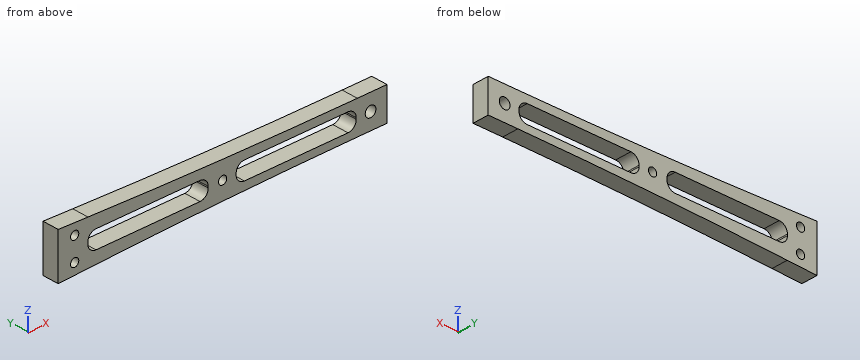
from build123d import *

# Parameters (mm, degrees)
SZKIC1_R                    = 1.97098021
SZKIC1_R_2                  = 3.25
SZKIC1_R_3                  = 2.5
DODANIE_WYCI_GNI_CIE1_DEPTH = 10
ZAOKR_GLENIE1_R             = 4100
OTW_R_GWINTOWANY_M62_D      = 5
OTW_R_GWINTOWANY_M62_DEPTH  = 15.497848452
OTW_R_GWINTOWANY_M62_TIP    = 1.502151548


with BuildPart() as part:
    # Szkic1 → Dodanie-wyciągnięcie1 (new body)
    with BuildSketch(Plane(origin=(0, 0, 0), x_dir=(1, 0, 0), z_dir=(0, 1, 0))):
        Polygon((200, 0), (200, 20), (100, 20), (0, 24), (0, -4), (100, 0), align=None)
        with Locations(Location((100, 10, 0), (0, 0, 270))):
            Circle(SZKIC1_R, mode=Mode.SUBTRACT)
        with Locations(Location((190, 10, 0), (0, 0, 270))):
            Circle(SZKIC1_R_2, mode=Mode.SUBTRACT)
        with Locations(Location((10, 17, 0), (0, 0, 270))):
            Circle(SZKIC1_R_3, mode=Mode.SUBTRACT)
        with Locations(Location((10, 3, 0), (0, 0, 270))):
            Circle(SZKIC1_R_3, mode=Mode.SUBTRACT)
        with BuildLine():
            Line((22.984822323, 15.57457628), (86.25939238, 15.57457628))
            ThreePointArc((86.25939238, 15.57457628), (89.794926286, 14.110110186), (91.25939238, 10.57457628))
            Line((91.25939238, 10.57457628), (91.25939238, 9.696719379))
            ThreePointArc((91.25939238, 9.696719379), (89.794926286, 6.161185473), (86.25939238, 4.696719379))
            Line((86.25939238, 4.696719379), (22.984822323, 4.696719379))
            ThreePointArc((22.984822323, 4.696719379), (19.449288417, 6.161185473), (17.984822323, 9.696719379))
            Line((17.984822323, 9.696719379), (17.984822323, 10.57457628))
            ThreePointArc((17.984822323, 10.57457628), (19.449288417, 14.110110186), (22.984822323, 15.57457628))
        make_face(mode=Mode.SUBTRACT)
        with BuildLine():
            Line((113.225148066, 15.57457628), (176.286209663, 15.57457628))
            ThreePointArc((176.286209663, 15.57457628), (179.821743569, 14.110110186), (181.286209663, 10.57457628))
            Line((181.286209663, 10.57457628), (181.286209663, 9.752776346))
            ThreePointArc((181.286209663, 9.752776346), (179.821743569, 6.21724244), (176.286209663, 4.752776346))
            Line((176.286209663, 4.752776346), (113.225148066, 4.752776346))
            ThreePointArc((113.225148066, 4.752776346), (109.68961416, 6.21724244), (108.225148066, 9.752776346))
            Line((108.225148066, 9.752776346), (108.225148066, 10.57457628))
            ThreePointArc((108.225148066, 10.57457628), (109.68961416, 14.110110186), (113.225148066, 15.57457628))
        make_face(mode=Mode.SUBTRACT)
    extrude(amount=DODANIE_WYCI_GNI_CIE1_DEPTH)

    # Zaokrąglenie1
    # the kernel refuses this fillet: 4100 mm, written as the material it adds along each edge
    with BuildSketch(Plane(origin=(100, 0, -20), x_dir=(1, 0, 0), z_dir=(0, 1, 0)), Plane(origin=(100, 0, 0), x_dir=(-0.9992009587217893, 0, 0.03996803834887583), z_dir=(0, 1, 0))) as zaokr_glenie1_piece_1:
        with BuildLine():
            CenterArc((ZAOKR_GLENIE1_R * 0.0199920063936, ZAOKR_GLENIE1_R), ZAOKR_GLENIE1_R, 267.709389957, 2.290610043)
            Line((-ZAOKR_GLENIE1_R * 0.0199760319553, ZAOKR_GLENIE1_R * 0.000799041278211), (0, 0))
            Line((0, 0), (ZAOKR_GLENIE1_R * 0.0199920063936, 0))
        make_face()
    extrude(amount=10)

    # Otwór gwintowany M62
    with Locations(Plane(origin=(100, 10, -10), x_dir=(0, 0, 1), z_dir=(0, 1, 0))):
        with Locations((0, 0)):
            Hole(OTW_R_GWINTOWANY_M62_D / 2, depth=OTW_R_GWINTOWANY_M62_DEPTH)
            with Locations((0, 0, -(OTW_R_GWINTOWANY_M62_DEPTH + OTW_R_GWINTOWANY_M62_TIP / 2))):  # 118° drill point
                Cone(0, OTW_R_GWINTOWANY_M62_D / 2, OTW_R_GWINTOWANY_M62_TIP, mode=Mode.SUBTRACT)


solid = part.part
Geometry check sheet. Reference: the model listing, model coordinates, mm. Give positions to 0.01 mm unless a question says otherwise; leave off trailing zeros. Loops run counter-clockwise (first coordinate to the right, second up) from the corner with the lowest first, then second, coordinate; pieces in that order, holes last. Notation, with made-up numbers: M -26,35 L 12,35 A16 cw 12,57 Z; hole C -39.5,4.25 d2. An arc over 180 degrees is marked long. Answer as a JSON object with one key per item and string values. Group by question number.
Item 1: Material ranges on L1, parallel to X at y = 2.5, z = -10; L2, parallel to X at y = 5.5, z = -3; L3, parallel to X at y = 4.75, z = -5.25, recorded low to high.
Item 2: Sectioned sample at C-C on y = 3.25. Record the boundary of the cut face in (x, z), plus the area to 3 significant figures.
Item 3: Sectioned sample at A-A on x = 178. Record the boundary of the cut face in (y, z), plus the area to 3 significant figures.
Item 4: Sectioned sample at D-D on x = 10. Record the boundary of the cut face in (y, z).
Item 5: Sectioned sample at B-B on z = -3. Record the boundary of the cut face in (x, y), plus the area to 3 significant figures.
Item 6: Gauge pin test, flat ends, axial feed: pin 1 (5 mm diameter, centred on x = 188, y = 2.5, fed in from -Z); pin 2 (5 mm diameter, centred on x = 133.5, y = 7.5, fed in from -Z). Record the tip position at first contact, or that the pin passes through.
Findings below:
{
 "1": {"L1": "0 to 17.98, 91.26 to 97.5, 102.5 to 108.23, 181.29 to 186.75, 193.25 to 200", "L2": "0 to 7.5, 12.5 to 200", "L3": "0 to 8.91, 11.09 to 20.7, 88.55 to 111.05, 178.46 to 200"},
 "2": {"outline": "M 0,-24 L 18.1,-23.28 A4100 cw 181.97,-20 L 200,-20 L 200,0 L 181.97,0 A4100 cw 18.1,3.28 L 0,4 Z; hole C 10,-17 d5; hole C 10,-3 d5; hole M 17.98,-10.57 A5 ccw 22.98,-15.57 L 86.26,-15.57 A5 ccw 91.26,-10.57 L 91.26,-9.7 A5 ccw 86.26,-4.7 L 22.98,-4.7 A5 ccw 17.98,-9.7 Z; hole C 100,-10 d5; hole M 108.23,-10.57 A5 ccw 113.23,-15.57 L 176.29,-15.57 A5 ccw 181.29,-10.57 L 181.29,-9.75 A5 ccw 176.29,-4.75 L 113.23,-4.75 A5 ccw 108.23,-9.75 Z; hole C 190,-10 d6.5", "area": "2,850 mm2"},
 "3": {"outline": "M 0,-20 L 10,-20 L 10,-15.27 L 0,-15.27 Z; M 0,-5.06 L 10,-5.06 L 10,0 L 0,0 Z", "area": "97.9 mm2"},
 "4": {"outline": "M 0,-23.6 L 10,-23.6 L 10,-19.5 L 0,-19.5 Z; M 0,-14.5 L 10,-14.5 L 10,-5.5 L 0,-5.5 Z; M 0,-0.5 L 10,-0.5 L 10,3.6 L 0,3.6 Z"},
 "5": {"outline": "M 0,0 L 7.5,0 L 7.5,10 L 0,10 Z; M 12.5,0 L 200,0 L 200,10 L 12.5,10 Z", "area": "1,950 mm2"},
 "6": {"pin 1": "z = -20", "pin 2": "z = -20.32"}
}
